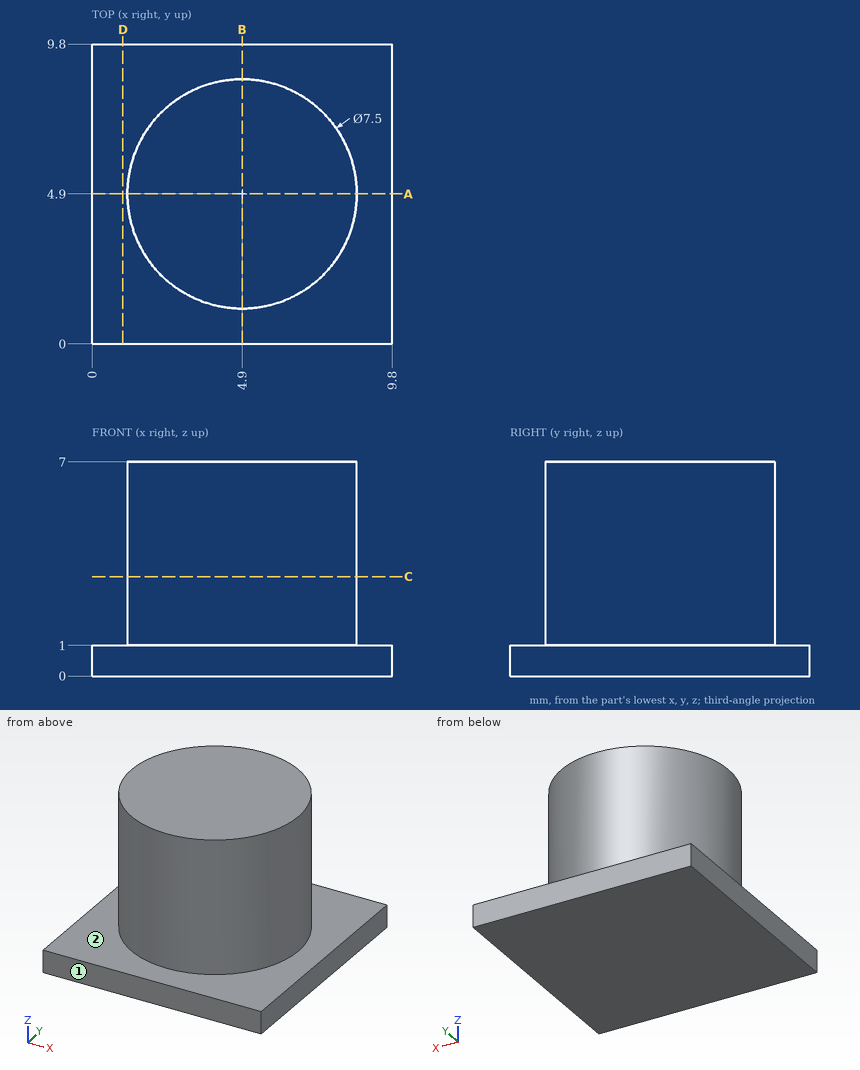
Geometry check sheet. Reference: drawing and pictorial views, mm from the part's lowest x, y, z. A direction names the side the tool comes from. Round coordinates to 2 decimals unless told otherwise and drop trailing zeros. Loops run counter-clockwise (first coordinate to the right, second up) from the corner with the lowest first, then second, coordinate; pieces in that order, holes last.
1. Sectioned sample at C-C on z = 3.25. Record the boundary of the cut face in (x, y).
2. Gauge pin test, flat ends, axial feed: pin 1 Ø3 at (y, z) = (3, 5.5) entering from -X; pin 2 Ø4 at (x, z) = (5, 5) entering from +Y. Record the tip position at first contact, or that the pin passes through.
3. Sectioned sample at A-A on y = 4.9. Record the boundary of the cut face in (x, z), and give its area (3 significant figures).
4. Sectioned sample at D-D on x = 1. Record the boundary of the cut face in (y, z), and give its area (3 significant figures).
5. Set-up check for the marked faces 1 and 2: record each of +Z, -Z, +X, -X, +Y, -Y from which the full face is reachable in a straight line by a thin tool's end or side.
6. Scan lines: probe 1 along Z at (x, y) = (9.25, 6.5); probe 2 along Y at (x, z) = (3.75, 1.25); probe 3 along X at (y, z) = (8.25, 2). Record each from-to range of solid material in increasing order.
Recorded:
1. outline: circle Ø7.5 at (4.9, 4.9)
2. pin 1: stops at x = 1.17
2. pin 2: stops at y = 8.65
3. outline: (0, 0) - (9.8, 0) - (9.8, 1) - (8.65, 1) - (8.65, 7) - (1.15, 7) - (1.15, 1) - (0, 1) - close
3. area: 54.8 mm2
4. outline: (0, 0) - (9.8, 0) - (9.8, 1) - (0, 1) - close
4. area: 9.80 mm2
5. face 1: +Z, -Z, +X, -X, -Y
5. face 2: +Z
6. probe 1: z = 0 to 1
6. probe 2: y = 1.33 to 8.47
6. probe 3: x = 3.21 to 6.59
